Autodesk Inventor part; units mm, degrees
ref_plane "Work Plane1" through (24.13, 24.13, 0) normal (0, 0, -1) x (-1, 0, 0)
ref_plane "Work Plane2" through (24.13, 24.13, 0) normal (0, 0, 1) x (1, 0, 0)
ref_plane "YZ Plane" through (0, 0, 0) normal (1, 0, 0) x (0, 1, 0)
ref_plane "Work Plane1" through (24.13, 24.13, 0) normal (0, 0, -1) x (-1, 0, 0)
sketch "Sketch1" plane through (24.13, 24.13, 0) normal (0, 0, -1) x (-1, 0, 0)
  line L0 (0, 0) -> (21.59, 0)
  line L1 (-2.54, -21.59) -> (-2.54, -2.54)
  line L2 (-2.54, -2.54) -> (-2.54, 0)
  line L3 (-2.54, 0) -> (0, 0)
  line L4 (24.13, -24.13) -> (-2.54, -24.13)
  line L5 (-2.54, -24.13) -> (-2.54, 0)
  line L6 (-2.54, 0) -> (24.13, 0)
  line L7 (24.13, 0) -> (24.13, -24.13)
  line L8 (10.795, -24.13) -> (10.414, 0)
  line L9 (24.13, -12.065) -> (10.6045, -12.065)
  line L10 (-33.5455, 0) -> (54.7545, 0)
  line L11 (54.7545, 0) -> (54.7545, -24.13)
  line L12 (54.7545, -24.13) -> (-33.5455, -24.13)
  line L13 (-33.5455, -24.13) -> (-33.5455, 0)
  line L14 (-33.5455, 0) -> (54.7545, -24.13) construction
  line L15 (54.7545, 0) -> (-33.5455, -24.13) construction
  dimension "d1" = 88.3
extrude "Extrusion1" add sketch "Sketch1" along normal blind 4
sketch "Sketch2" plane through (24.13, 24.13, 0) normal (0, 0, 1) x (1, 0, 0)
  circle A0 centre (-21.59, -17.145) radius 1.1
  circle A1 centre (-21.59, -17.145) radius 1.1
  circle A2 centre (0, -17.145) radius 1.1
  circle A3 centre (0, -17.145) radius 1.1
  circle A4 centre (0, -2.54) radius 1.1
  circle A5 centre (0, -2.54) radius 1.1
  circle A6 centre (-21.59, -2.54) radius 1.1
  circle A7 centre (-21.59, -2.54) radius 1.1
  point P0 (-24.13, -24.13)
extrude "Extrusion2" cut sketch "Sketch2" against normal blind 4
ref_plane "Work Plane2" through (24.13, 24.13, 0) normal (0, 0, 1) x (1, 0, 0)
sketch "Sketch3" plane through (24.13, 24.13, 0) normal (0, 0, 1) x (1, 0, 0)
  line L0 (-54.7545, -24.13) -> (-54.7545, 0)
  line L1 (-54.7545, -12.065) -> (-44.7545, -12.065)
  line L2 (33.5455, 0) -> (33.5455, -24.13)
  line L3 (33.5455, -12.065) -> (23.5455, -12.065)
  circle A0 centre (-44.7545, -12.065) radius 2.5
  circle A1 centre (23.5455, -12.065) radius 2.5
  point P0 (-24.13, -24.13)
  dimension "d6" = 10
  dimension "d7" = 10
  dimension "d8" = 5
  dimension "d9" = 5
extrude "Extrusion3" cut sketch "Sketch3" against normal blind 4
properties part number "A4988_driver_holder"
The model under review builds one solid part; all positions refer to its coordinate system, in mm. Give positions to 0.01 mm unless a question says otherwise; leave off trailing zeros. Write each loop counter-clockwise with the first axis right and the second up, starting at its lowest first coordinate (ties: lowest second). Pieces come first, ordered by that corner, then holes. Notation, with made-up numbers: M 34,-13 L 50,-13 A21 cw 50,16 Z; hole C 15.25,82.25 d2. An arc over 180 degrees is marked long. Write each question's results on one line, items separated by ' | '. Start each with the question number.
1. We need section A-A (y = 21.59). Write out the cut boundary in (x, z), and give its area (3 significant figures).
2. For probe 1 along Y at (x, z) = (2.54, -1) (3 decimals); probe 2 along X at (y, z) = (12, -0.65); probe 3 along X at (y, z) = (13.75, -1.75), list the stretches that pass through material, from the lowest coordinate up. Write a range as [from, to].
3. We need section C-C (z = -2.05). Write out the cut boundary in (x, y) (1 decimal).
4. Mouldability with a two-part tool opening along Y and no side actions: class faces 1 (the flat face through (14, 12, -4)), 2 (the cylindrical face through (45.178, 12.175, -1.972)), 3 (the flat face through (13, 0, -2)) as released by +Y, released by -Y, zero draft, split by the parting line, or undercut.
5. We need section B-B (x = 24.13). Write out the cut boundary in (y, z) (3 decimals).
Results found:
1) outline: M -30.62,-4 L 1.44,-4 L 1.44,0 L -30.62,0 Z; M 3.64,-4 L 23.03,-4 L 23.03,0 L 3.64,0 Z; M 25.23,-4 L 57.68,-4 L 57.68,0 L 25.23,0 Z | area: 336 mm^2
2) probe 1: y = [0, 5.885], [8.085, 20.49], [22.69, 24.13] | probe 2: x = [-30.62, -23.12], [-18.13, 45.18], [50.17, 57.68] | probe 3: x = [-30.62, -22.47], [-18.78, 45.83], [49.52, 57.68]
3) outline: M -30.6,0 L 57.7,0 L 57.7,24.1 L -30.6,24.1 Z; hole C -20.6,12.1 d5; hole C 2.5,7 d2.2; hole C 2.5,21.6 d2.2; hole C 24.1,7 d2.2; hole C 24.1,21.6 d2.2; hole C 47.7,12.1 d5
4) face 1: zero draft | face 2: undercut | face 3: released by -Y
5) outline: M 0,-4 L 5.885,-4 L 5.885,0 L 0,0 Z; M 8.085,-4 L 20.49,-4 L 20.49,0 L 8.085,0 Z; M 22.69,-4 L 24.13,-4 L 24.13,0 L 22.69,0 Z
